from build123d import *

# Parameters (mm, degrees)
SKETCH1_W                        = 254
SKETCH1_H                        = 438.15
BOSS_EXTRUDE1_DEPTH              = 6.35
F_27_64_0_42188_DIAMETER_HOLE1_D = 10.715752
SKETCH4_W                        = 254
SKETCH4_H                        = 12.7
BOSS_EXTRUDE2_DEPTH              = 6.35
FILLET1_R                        = 2.54


with BuildPart() as part:
    # Sketch1 → Boss-Extrude1 (new body)
    with BuildSketch(Plane(origin=(0, 0, 0), x_dir=(0, 0, -1), z_dir=(1, 0, 0))):
        with Locations((127, 219.075)):
            Rectangle(SKETCH1_W, SKETCH1_H)
    extrude(amount=BOSS_EXTRUDE1_DEPTH)

    # 27/64 (0.42188) Diameter Hole1 (through all)
    with Locations(Plane(origin=(6.35, 0, 0), x_dir=(0, 0, -1), z_dir=(1, 0, 0))):
        with Locations((25.4, 412.75), (25.4, 219.075), (228.6, 219.075), (228.6, 412.75)):
            Hole(F_27_64_0_42188_DIAMETER_HOLE1_D / 2)

    # Sketch4 → Boss-Extrude2 (add)
    with BuildSketch(Plane(origin=(6.35, 0, 0), x_dir=(0, 0, -1), z_dir=(1, 0, 0))):
        with Locations((127, 444.5)):
            Rectangle(SKETCH4_W, SKETCH4_H)
    extrude(amount=-BOSS_EXTRUDE2_DEPTH)

    # Fillet1
    fillet1_edges = [part.edges().sort_by_distance(p)[0] for p in [
        (3.175, 450.85, -254),
        (3.175, 450.85, 0),
        (3.175, 0, -254),
        (3.175, 0, 0),
    ]]
    fillet(fillet1_edges, radius=FILLET1_R)


solid = part.part
Here's how the part is built. I have some questions about the finished solid (model axes, mm). Round coordinates to 2 decimals unless told otherwise and drop trailing zeros. Order: outer loops, then holes, each group sorted by start corner. A loop starts at its lowest first (then second) coordinate and runs counter-clockwise, first axis right, second up. Notation, with made-up numbers: M -37,70.25 L 9,70.25 A14 cw 9,87.25 Z; hole C 82.25,35.25 d6. An arc over 180 degrees is marked long. Return JSON: item names as keys, results as strings. Group by question number.
1. Please list where these lines run through material, in increasing order: probe 1 along Z at (x, y) = (3.75, 412.75); probe 2 along Y at (x, z) = (2, -25.4).
2. If we section it at B-B on y = 412.75: List the corners of the cut face in (x, z) for me, then the cut area to 3 significant figures.
3. If we section it at A-A on z = -25.4: List the corners of the cut face in (x, y) for me.
4. If we mould it in two halves opening along Y, with no side actions, what happens to faces 1 (the face through (3.13, 418.06, -26.1)), 2 (the face through (0, 229, -125))? For each: pulls with the +Y half, pulls with the -Y half, needs draft (parallel to the pull), parting line crosses it, or undercut.
Reply:
{
 "1": {"probe 1": "-254 to -233.96, -223.24 to -30.76, -20.04 to 0", "probe 2": "0 to 213.72, 224.43 to 407.39, 418.11 to 450.85"},
 "2": {"outline": "M 0,-254 L 6.35,-254 L 6.35,-233.96 L 0,-233.96 Z; M 0,-223.24 L 6.35,-223.24 L 6.35,-30.76 L 0,-30.76 Z; M 0,-20.04 L 6.35,-20.04 L 6.35,0 L 0,0 Z", "area": "1,480 mm^2"},
 "3": {"outline": "M 0,0 L 6.35,0 L 6.35,213.72 L 0,213.72 Z; M 0,224.43 L 6.35,224.43 L 6.35,407.39 L 0,407.39 Z; M 0,418.11 L 6.35,418.11 L 6.35,450.85 L 0,450.85 Z"},
 "4": {"face 1": "undercut", "face 2": "needs draft"}
}
